from build123d import *

# Parameters (mm, degrees)
SKETCH2_R           = 5
BOSS_EXTRUDE1_DEPTH = 20
SKETCH4_R           = 4
CUT_EXTRUDE1_DEPTH  = 26


with BuildPart() as part:
    # Sketch2 → Boss-Extrude1 (new body)
    with BuildSketch(Plane.XY):
        with BuildLine():
            Line((-10, -50), (-10, 50))
            ThreePointArc((-10, 50), (0, 60), (10, 50))
            Line((10, 50), (10, -50))
            ThreePointArc((10, -50), (0, -60), (-10, -50))
        make_face()
        with Locations((0, -50)):
            Circle(SKETCH2_R, mode=Mode.SUBTRACT)
    extrude(amount=BOSS_EXTRUDE1_DEPTH)

    # Sketch4 → Cut-Extrude1 (cut)
    with BuildSketch(Plane(origin=(10, 0, 0), x_dir=(0, 0, -1), z_dir=(1, 0, 0))):
        with Locations(Location((-10, 43.355409554, 0), (0, 0, 90))):
            Circle(SKETCH4_R)
    extrude(amount=-CUT_EXTRUDE1_DEPTH, mode=Mode.SUBTRACT)


solid = part.part
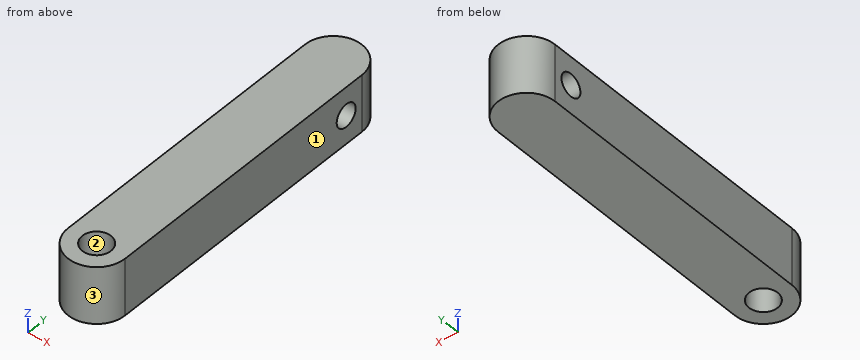
Can you work these out from the model? Positions are in its coordinate system, mm. Face numbers are marked on the shaded views. Coordinates: 2 decimals unless noted, no trailing zeros. Write each loop counter-clockwise with the first axis right and the second up, starting at its lowest first coordinate (ties: lowest second). Pieces come first, ordered by that corner, then holes. Notation, with made-up numbers: M -25.5,-15.5 L -8.5,-15.5 A20 ccw -8.5,11.5 Z; hole C 70,83 d7. An arc over 180 degrees is marked long. Use one line per item in the form item = value.
Q1. If we section it at B-B (z = 10): Write out the boundary of the cut face in (x, y).
Model answer:
outline = M -10,-50 A10 ccw 10,-50 L 10,39.36 L -10,39.36 Z; M -10,47.36 L 10,47.36 L 10,50 A10 ccw -10,50 Z; hole C 0,-50 d10
Q2. If we section it at D-D (x = 8.5): Write out the boundary of the cut face in (y, z), then the cut area to 3 significant figures.
Model answer:
outline = M -55.27,0 L 55.27,0 L 55.27,20 L -55.27,20 Z; hole C 43.36,10 d8
area = 2,160 mm^2
Q3. We'd pull the mould along X, two halves only. Please class the marked faces 1, 2 and 3: +X half, -X half, draft (parallel to the pull), parting line (faces both ways), or undercut.
Model answer:
face_1 = +X half
face_2 = undercut
face_3 = parting line
Q4. I need wall thicknesses on line 1 along Y through (x, z) = (0, 17); line 2 along Y through (x, z) = (0, 13.25); line 3 along Y through (x, z) = (0, 12.75). Which ranges of each line are inside material? Lowest first, please. Write a range as from..to.
Model answer:
line_1 = -60..-55, -45..60
line_2 = -60..-55, -45..41.02, 45.69..60
line_3 = -60..-55, -45..40.45, 46.26..60
Q5. If we section it at A-A (x = 0): Write out the boundary of the cut face in (y, z).
Model answer:
outline = M -60,0 L -55,0 L -55,20 L -60,20 Z; M -45,0 L 60,0 L 60,20 L -45,20 Z; hole C 43.36,10 d8
Q6. If we section it at C-C (y = 43): Write out the boundary of the cut face in (x, z), then the cut area to 3 significant figures.
Model answer:
outline = M -10,0 L 10,0 L 10,6.02 L -10,6.02 Z; M -10,13.98 L 10,13.98 L 10,20 L -10,20 Z
area = 241 mm^2
Q7. For P1, Ø10, axis at x = 6.5, z = 9, coming from the -Y side; P2, Ø12, axis at x = 6, y = 42.5, coming from the -Z side; P3, Ø6, axis at x = 0, y = -50, coming from the +Z side, each with a flat end and sliding along its axis, tell me the tip position at first contact or that it passes through.
Model answer:
P1 = -59.89
P2 = 0
P3 = through
